Geometry check sheet. Reference: the model listing, model coordinates, mm. A direction names the side the tool comes from. Coordinates: 2 decimals unless noted, no trailing zeros. Write each loop counter-clockwise with the first axis right and the second up, starting at its lowest first coordinate (ties: lowest second). Pieces come first, ordered by that corner, then holes. Notation, with made-up numbers: (3.5, 60.5) -> (54.5, 60.5) arc R14 ccw to (54.5, 68.5) -> close; hole circle Ø6 at (-8, 68). An arc over 180 degrees is marked (long way). One line per question, with ' | ' between items.
```python
from build123d import *

# Parameters (mm, degrees)
SKETCH1_W           = 55
SKETCH1_H           = 25
BOSS_EXTRUDE1_DEPTH = 16.5
CUT_EXTRUDE1_DEPTH  = 20
SKETCH3_W           = 51
SKETCH3_H           = 2.5
CUT_EXTRUDE2_DEPTH  = 2.5
SKETCH4_W           = 41
SKETCH4_H           = 3
BOSS_EXTRUDE2_DEPTH = 15
SKETCH5_W           = 46.5
SKETCH5_H           = 6
CUT_EXTRUDE3_DEPTH  = 15


with BuildPart() as part:
    # Sketch1 → Boss-Extrude1 (new body)
    with BuildSketch(Plane.XY):
        with Locations((27.5, 12.5)):
            Rectangle(SKETCH1_W, SKETCH1_H)
    extrude(amount=BOSS_EXTRUDE1_DEPTH)

    # Sketch2 → Cut-Extrude1 (cut)
    with BuildSketch(Plane(origin=(0, 25, 0), x_dir=(1, 0, 0), z_dir=(0, 1, 0))):
        Polygon((2, -12), (4, -12), (4, -2), (50.5, -2), (50.5, -12), (53, -12), (53, -14.5), (50.5, -14.5), (50.5, -16.5), (4, -16.5), (4, -14.5), (2, -14.5), align=None)
    extrude(amount=-CUT_EXTRUDE1_DEPTH, mode=Mode.SUBTRACT)

    # Sketch3 → Cut-Extrude2 (cut)
    with BuildSketch(Plane(origin=(0, 5, 0), x_dir=(1, 0, 0), z_dir=(0, 1, 0))):
        with Locations((27.5, -13.25)):
            Rectangle(SKETCH3_W, SKETCH3_H)
    extrude(amount=-CUT_EXTRUDE2_DEPTH, mode=Mode.SUBTRACT)

    # Sketch4 → Boss-Extrude2 (add)
    with BuildSketch(Plane(origin=(0, 0, 0), x_dir=(-1, 0, 0), z_dir=(0, 0, -1))):
        with Locations((-27.5, 1.5)):
            Rectangle(SKETCH4_W, SKETCH4_H)
    extrude(amount=BOSS_EXTRUDE2_DEPTH)

    # Sketch5 → Cut-Extrude3 (cut)
    with BuildSketch(Plane.XY.offset(2)):
        with Locations((27.25, 22)):
            Rectangle(SKETCH5_W, SKETCH5_H)
    extrude(amount=-CUT_EXTRUDE3_DEPTH, mode=Mode.SUBTRACT)


solid = part.part
```
(1) Material ranges on line 1 (Z direction, x = 27, y = 3.5); line 2 (X direction, y = 9.25, z = 10); line 3 (X direction, y = 16, z = 14), recorded low to high.
Answers below:
line 1: z = 0 to 12, 14.5 to 16.5 | line 2: x = 0 to 4, 50.5 to 55 | line 3: x = 0 to 2, 53 to 55
(2) Depth check by flat-ended pin: P1, Ø5, axis at x = 8, y = 19, coming from the +Z side; P2, Ø0.6, axis at x = 31, z = 15.5, coming from the +Y side; P3, Ø2.5, axis at y = 1.5, z = -7.5, coming from the +X side. Enter the tip coordinate at first touch or a pass-through.
Answers below:
P1: stops at z = 2 | P2: stops at y = 5 | P3: stops at x = 48
(3) Draft check along Z on faces 1 (the face through (53, 14, 13)), 2 (the face through (28, 5, 7)), 3 (the face through (28, 2, -15)). Enter one of: pulls with the +Z half, pulls with the -Z half, needs draft (parallel to the pull), parting line crosses it, or undercut.
Answers below:
face 1: undercut | face 2: needs draft | face 3: pulls with the -Z half
(4) Cross-section at D-D (x = 22.5). Record the cut outline in (y, z).
Answers below:
outline: (0, -15) -> (3, -15) -> (3, 0) -> (19, 0) -> (19, 2) -> (5, 2) -> (5, 12) -> (2.5, 12) -> (2.5, 14.5) -> (5, 14.5) -> (5, 16.5) -> (0, 16.5) -> close
(5) Tool access check on faces 4 (the face through (27, 19, 1)), 5 (the face through (28, 4, 14.5)), 6 (the face through (7, 1, -7)), 7 (the face through (48, 1, -7)), 8 (the face through (4, 15, 6)). Record the directions out of +Z, -Z, +X, -X, +Y, -Y that give a thin tool (end or side, any length) a straight path to the whole face; none if there is none.
Answers below:
face 4: +Z, -Z, +Y | face 5: +Y | face 6: -Z, -X, +Y, -Y | face 7: -Z, +X, +Y, -Y | face 8: +Z, +Y
(6) Cross-section at A-A (y = 21.5). Record the cut outline in (x, z).
Answers below:
outline: (0, 0) -> (4, 0) -> (4, 12) -> (2, 12) -> (2, 14.5) -> (4, 14.5) -> (4, 16.5) -> (0, 16.5) -> close; (50.5, 0) -> (55, 0) -> (55, 16.5) -> (50.5, 16.5) -> (50.5, 14.5) -> (53, 14.5) -> (53, 12) -> (50.5, 12) -> close
(7) Cross-section at B-B (y = 16.25). Record the cut outline in (x, z), plus the area to 3 significant figures.
Answers below:
outline: (0, 0) -> (55, 0) -> (55, 16.5) -> (50.5, 16.5) -> (50.5, 14.5) -> (53, 14.5) -> (53, 12) -> (50.5, 12) -> (50.5, 2) -> (4, 2) -> (4, 12) -> (2, 12) -> (2, 14.5) -> (4, 14.5) -> (4, 16.5) -> (0, 16.5) -> close | area: 222 mm²
(8) Cross-section at C-C (z = 11). Record the cut outline in (x, y), plus the area to 3 significant figures.
Answers below:
outline: (0, 0) -> (55, 0) -> (55, 25) -> (50.5, 25) -> (50.5, 5) -> (4, 5) -> (4, 25) -> (0, 25) -> close | area: 445 mm²
